Could you check a few things on this model? Use its own coordinates, in mm. A direction names the side the tool comes from. Coordinates: 2 decimals unless noted, no trailing zeros. Order: outer loops, then holes, each group sorted by start corner. A loop starts at its lowest first (then second) coordinate and runs counter-clockwise, first axis right, second up. Notation, with made-up numbers: (53.5, 25.25) -> (97.5, 25.25) arc R16 cw to (97.5, 56.25) -> close; hole circle Ø8 at (85, 68). An arc over 180 degrees is marked (long way). Use a Markdown table: item, result. Add a question column.
1) If we section it at C-C (z = -10): Write out the boundary of the cut face in (x, y), plus the area to 3 significant figures.
2) If we section it at B-B (x = 80): Write out the boundary of the cut face in (y, z).
3) If we section it at D-D (y = 77): Write out the boundary of the cut face in (x, z), plus the area to 3 significant figures.
4) If we section it at A-A (y = 51): Write out the boundary of the cut face in (x, z).
5) Which directions (+Z, -Z, +X, -X, +Y, -Y) give clear straight access to the entire face, cutting with the end or side of a thin tool? Please do faces 1 (the flat face through (144, 96.8, -7)), 2 (the flat face through (144, 50, 0)).
6) Will these pins go through, and if not, where does the flat tip stop? pin 1 Ø4 at (x, y) = (48, 28) entering from -Z; pin 2 Ø6 at (x, y) = (167.5, 27) entering from +Z.
7) If I drill on L1, parallel to Y at x = 275.5, z = -9.5; L2, parallel to Y at x = 281, z = -0.8; L3, parallel to Z at x = 73, y = 58.5, over which ranges is the centre line in solid material (lowest first)? Write a range as [from, to].
```python
from build123d import *

# Parameters (mm, degrees)
SKETCH_1_W                         = 292
SKETCH_1_H                         = 98
SKETCH_1_R                         = 2
SM_BASE_FLANGE_1_DEPTH             = 1.2
SM_EDGE_FLANGE_1_STRIP_W           = 6.2732
SM_EDGE_FLANGE_1_STRIP_H           = 1.2
SM_EDGE_FLANGE_1_STRIP_CUT_DEPTH   = 292
SM_EDGE_FLANGE_1_STRIP_2_W         = 6.2732
SM_EDGE_FLANGE_1_STRIP_2_H         = 1.2
SM_EDGE_FLANGE_1_STRIP_CUT_2_DEPTH = 292
SM_EDGE_FLANGE_1_DEPTH             = 292
SM_EDGE_FLANGE_1_BEND_DEPTH        = 292
CUT_EXTRUDE_1_DEPTH                = 309.240166104


# Sheet-metal steps are written as plain solids
with BuildPart() as part:
    # Sketch 1 → Базовая кромка1 (new body)
    with BuildSketch(Plane.XY):
        with Locations((146, 49)):
            Rectangle(SKETCH_1_W, SKETCH_1_H)
        with Locations((281, 86)):
            Circle(SKETCH_1_R, mode=Mode.SUBTRACT)
        with Locations((281, 71)):
            Circle(SKETCH_1_R, mode=Mode.SUBTRACT)
        with Locations((281, 27)):
            Circle(SKETCH_1_R, mode=Mode.SUBTRACT)
        with Locations((281, 12)):
            Circle(SKETCH_1_R, mode=Mode.SUBTRACT)
        with BuildLine():
            Line((21.75, 54.196152423), (21.75, 43.803847577))
            ThreePointArc((21.75, 43.803847577), (30, 39.25), (38.25, 43.803847577))
            Line((38.25, 43.803847577), (38.25, 54.196152423))
            ThreePointArc((38.25, 54.196152423), (30, 58.75), (21.75, 54.196152423))
        make_face(mode=Mode.SUBTRACT)
    extrude(amount=-SM_BASE_FLANGE_1_DEPTH)

    # Ребро-кромка1 strip (across the edge) → Ребро-кромка1 strip cut (cut)
    with BuildSketch(Plane(origin=(0, 98, -1.2), x_dir=(0, -1, 0), z_dir=(1, 0, 0))):
        with Locations((-1.2, -0.6)):
            Rectangle(SM_EDGE_FLANGE_1_STRIP_W, SM_EDGE_FLANGE_1_STRIP_H)
    extrude(amount=SM_EDGE_FLANGE_1_STRIP_CUT_DEPTH, mode=Mode.SUBTRACT)

    # Ребро-кромка1 strip 2 (across the edge) → Ребро-кромка1 strip cut 2 (cut)
    with BuildSketch(Plane(origin=(292, 0, -1.2), x_dir=(0, 1, 0), z_dir=(-1, 0, 0))):
        with Locations((-1.2, -0.6)):
            Rectangle(SM_EDGE_FLANGE_1_STRIP_2_W, SM_EDGE_FLANGE_1_STRIP_2_H)
    extrude(amount=SM_EDGE_FLANGE_1_STRIP_CUT_2_DEPTH, mode=Mode.SUBTRACT)

    # Ребро-кромка1 section (across the edge) → Ребро-кромка1 (add)
    with BuildSketch(Plane(origin=(0, 98, -1.2), x_dir=(0, -1, 0), z_dir=(1, 0, 0))):
        with BuildLine():
            Line((0, 0.7366), (0, 10.8))
            Line((0, 10.8), (1.2, 10.8))
            Line((1.2, 10.8), (1.2, 0.7366))
            ThreePointArc((1.2, 0.7366), (1.415745145, 0.215745145), (1.9366, 0))
            Line((1.9366, 0), (1.9366, -1.2))
            ThreePointArc((1.9366, -1.2), (0.567217008, -0.632782992), (0, 0.7366))
        make_face()
    extrude(amount=SM_EDGE_FLANGE_1_DEPTH)

    # Ребро-кромка1 section 2 (across the edge) → Ребро-кромка1 bend (add)
    with BuildSketch(Plane(origin=(292, 0, -1.2), x_dir=(0, 1, 0), z_dir=(-1, 0, 0))):
        with BuildLine():
            Line((0, 0.7366), (0, 10.8))
            Line((0, 10.8), (1.2, 10.8))
            Line((1.2, 10.8), (1.2, 0.7366))
            ThreePointArc((1.2, 0.7366), (1.415745145, 0.215745145), (1.9366, 0))
            Line((1.9366, 0), (1.9366, -1.2))
            ThreePointArc((1.9366, -1.2), (0.567217008, -0.632782992), (0, 0.7366))
        make_face()
    extrude(amount=SM_EDGE_FLANGE_1_BEND_DEPTH)

    # Эскиз12 → Вырез-Вытянуть1 (cut, through all)
    with BuildSketch(Plane(origin=(0, 98, 0), x_dir=(1, 0, 0), z_dir=(0, 1, 0))):
        with BuildLine():
            Line((9, 12), (0, 12))
            Line((0, 12), (0, 3))
            ThreePointArc((0, 3), (2.636038969, 9.363961031), (9, 12))
        make_face()
        with BuildLine():
            Line((283, 12), (292, 12))
            Line((292, 12), (292, 3))
            ThreePointArc((292, 3), (289.363961031, 9.363961031), (283, 12))
        make_face()
    extrude(amount=-CUT_EXTRUDE_1_DEPTH, mode=Mode.SUBTRACT)


solid = part.part
```
Answer sheet:
| question | item | result |
|---|---|---|
| 1 | outline | (3.34, 0) -> (288.66, 0) -> (288.66, 1.2) -> (3.34, 1.2) -> close; (3.34, 96.8) -> (288.66, 96.8) -> (288.66, 98) -> (3.34, 98) -> close |
| 1 | area | 685 mm2 |
| 2 | outline | (0, -12) -> (1.2, -12) -> (1.2, -1.94) arc R0.74 cw to (1.94, -1.2) -> (96.06, -1.2) arc R0.74 cw to (96.8, -1.94) -> (96.8, -12) -> (98, -12) -> (98, -1.94) arc R1.94 ccw to (96.06, 0) -> (1.94, 0) arc R1.94 ccw to (0, -1.94) -> close |
| 3 | outline | (0, -1.2) -> (292, -1.2) -> (292, 0) -> (0, 0) -> close |
| 3 | area | 350 mm2 |
| 4 | outline | (0, -1.2) -> (21.75, -1.2) -> (21.75, 0) -> (0, 0) -> close; (38.25, -1.2) -> (292, -1.2) -> (292, 0) -> (38.25, 0) -> close |
| 5 | face 1 | -Z, +X, -X |
| 5 | face 2 | +Z, +X, -X, +Y, -Y |
| 6 | pin 1 | z = -1.2 |
| 6 | pin 2 | z = 0 |
| 7 | L1 | [0, 1.2], [96.8, 98] |
| 7 | L2 | [0.37, 10], [14, 25], [29, 69], [73, 84], [88, 97.63] |
| 7 | L3 | [-1.2, 0] |
